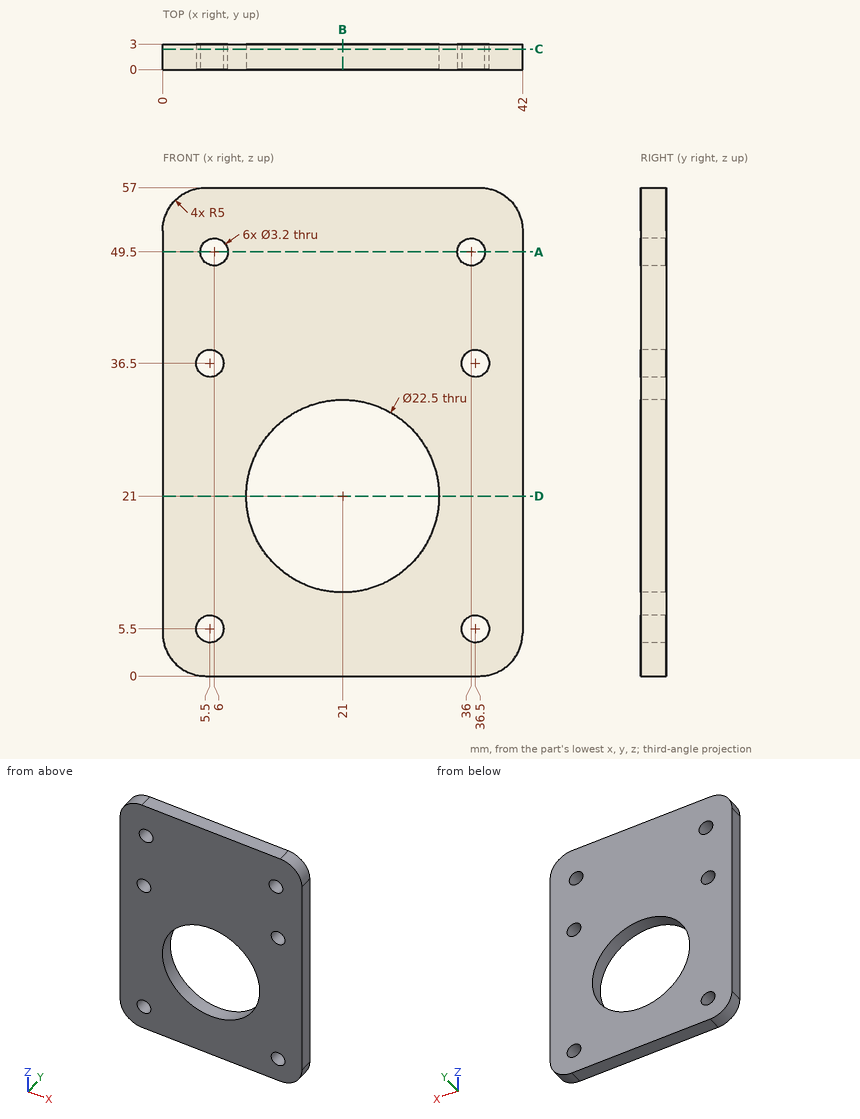
Geometry check sheet. Reference: drawing and pictorial views, mm from the part's lowest x, y, z. Give positions to 0.01 mm unless a question says otherwise; leave off trailing zeros. Write each loop counter-clockwise with the first axis right and the second up, starting at its lowest first coordinate (ties: lowest second). Pieces come first, ordered by that corner, then holes. Notation, with made-up numbers: (20, 73.5) -> (32, 73.5) arc R26 cw to (32, 109.5) -> close; hole circle Ø6 at (0, -11). An arc over 180 degrees is marked (long way). One line per item, written item: value. Start each with the question number.
Item 1: Section check D-D on z = 21. Record the cut outline in (x, y).
Item 2: Gauge pin test, flat end, axial feed: pin 1 (3 mm diameter, centred on x = 6, z = 49.5, fed in from -Y). Record the tip position at first contact, or that the pin passes through.
Item 3: Section check C-C on y = 2.4. Record the cut outline in (x, z).
Item 4: Section check A-A on z = 49.5. Record the cut outline in (x, y), then the cut area to 3 significant figures.
Item 5: Section check B-B on x = 21. Record the cut outline in (y, z), then the cut area to 4 significant figures.
Item 6: Material ranges on probe 1 along X at (y, z) = (1.35, 5.5); probe 2 along Z at (x, y) = (6, 2.1); probe 3 along Z at (x, y) = (36.5, 0.9), recorded low to high. Write a range as from..to.
Results list:
1. outline: (0, 0) -> (9.75, 0) -> (9.75, 3) -> (0, 3) -> close; (32.25, 0) -> (42, 0) -> (42, 3) -> (32.25, 3) -> close
2. pin 1: through
3. outline: (0, 5) arc R5 ccw to (5, 0) -> (37, 0) arc R5 ccw to (42, 5) -> (42, 52) arc R5 ccw to (37, 57) -> (5, 57) arc R5 ccw to (0, 52) -> close; hole circle Ø3.2 at (5.5, 5.5); hole circle Ø3.2 at (5.5, 36.5); hole circle Ø3.2 at (6, 49.5); hole circle Ø22.5 at (21, 21); hole circle Ø3.2 at (36, 49.5); hole circle Ø3.2 at (36.5, 5.5); hole circle Ø3.2 at (36.5, 36.5)
4. outline: (0, 0) -> (4.4, 0) -> (4.4, 3) -> (0, 3) -> close; (7.6, 0) -> (34.4, 0) -> (34.4, 3) -> (7.6, 3) -> close; (37.6, 0) -> (42, 0) -> (42, 3) -> (37.6, 3) -> close
4. area: 107 mm²
5. outline: (0, 0) -> (3, 0) -> (3, 9.75) -> (0, 9.75) -> close; (0, 32.25) -> (3, 32.25) -> (3, 57) -> (0, 57) -> close
5. area: 103.5 mm²
6. probe 1: 0..3.9, 7.1..34.9, 38.1..42
6. probe 2: 0..3.98, 7.02..34.98, 38.02..47.9, 51.1..57
6. probe 3: 0..3.9, 7.1..34.9, 38.1..47.98, 51.02..57
